Build history of the part. All positions in model axes, mm. A direction names the side the tool comes from. Round coordinates to 2 decimals unless told otherwise and drop trailing zeros. Write each loop counter-clockwise with the first axis right and the second up, starting at its lowest first coordinate (ties: lowest second). Pieces come first, ordered by that corner, then holes. Notation, with made-up numbers: (43, -12.5) -> (82, -12.5) arc R18 cw to (82, 11.5) -> close; hole circle Ø8 at (12.5, -2). An arc over 180 degrees is marked (long way). Answer in a Markdown table with one row per item. Add a question column.
from build123d import *

# Parameters (mm, degrees)
BOSS_EXTRUDE5_DEPTH      = 11
BOSS_EXTRUDE5_DEPTH_BACK = 5
SKETCH2_R                = 2.5


with BuildPart() as part:
    # Sketch1 → Revolve1 (revolve)
    with BuildSketch(Plane.XY, mode=Mode.PRIVATE) as revolve1_sk:
        Polygon((60, 80), (30, 80), (30, 40), (42.5, 40), (42.5, 0), (60, 0), align=None)
    revolve(revolve1_sk.sketch.rotate(Axis((30, 80, 0), (0, -1, 0)), 180), axis=Axis((30, 80, 0), (0, -1, 0)))

    # Sketch2 → Boss-Extrude5 (add, two sides: drawn at the far end of the back side and taken through both)
    with BuildSketch(Plane.XY.offset(-BOSS_EXTRUDE5_DEPTH_BACK)):
        with BuildLine():
            Line((46.5, 0), (46.5, -12))
            ThreePointArc((46.5, -12), (47.378679656, -14.121320344), (49.5, -15))
            Line((49.5, -15), (68.5, -15))
            ThreePointArc((68.5, -15), (70.621320344, -14.121320344), (71.5, -12))
            Line((71.5, -12), (71.5, -3))
            ThreePointArc((71.5, -3), (70.621320344, -0.878679656), (68.5, 0))
            Line((68.5, 0), (46.5, 0))
        make_face()
        with Locations((55, -8)):
            Circle(SKETCH2_R, mode=Mode.SUBTRACT)
    extrude(amount=BOSS_EXTRUDE5_DEPTH + BOSS_EXTRUDE5_DEPTH_BACK)


solid = part.part
(1) Saw through at A-A (y = -8). List the corners of the cut face in (x, z), plus the area to 3 significant figures.
(2) Drop flat-ended pins along their axis: P1, Ø16.5, axis at x = 60.5, y = -11, coming from the +Z side; P2, Ø4, axis at x = 59.5, z = -12.5, coming from the +Y side; P3, Ø3, axis at y = 38.5, z = -7.5, coming from the +X side; P4, Ø3, axis at x = 19, y = 25, coming from the +Z side. Give the stop position or say it passes through.
(3) Saw through at B-B (z = 0). List the corners of the cut face in (x, y), plus the area to 3 significant figures.
(4) Mould opens along Y. For faces 5 (the face through (57.31, -8.96, 2.89)), 6 (the face through (59, -7, 11)), 7 (the face through (30, 40, 0)) say: pulls with the +Y half, pulls with the -Y half, needs draft (parallel to the pull), parting line crosses it, or undercut.
(5) Probe line 1 along Y through (x, z) = (55, 1.5); line 2 along Z through (x, y) = (30, 31.5); line 3 along Z through (x, y) = (63, -0.5). List the from-to ranges inside material, lowest first.
(6) Which spindle directions (+Z, -Z, +X, -X, +Y, -Y) get a long thin tool onto all of the face, cutting with end or side? Do faces 1 (the face through (42.488, 19.72, -0.55)), 2 (the face through (46.5, -6, 3)), 3 (the face through (59, -7, -5)), 4 (the face through (70.6, -14.14, 2.89)). Say none if no direction does.
(7) Saw through at D-D (y = 11). List the corners of the cut face in (x, z), plus the area to 3 significant figures.
(8) Saw through at C-C (x = 30). List the corners of the cut face in (y, z).
Answer sheet:
| question | item | result |
|---|---|---|
| 1 | outline | (46.5, -5) -> (52.5, -5) -> (52.5, 11) -> (46.5, 11) -> close; (57.5, -5) -> (71.5, -5) -> (71.5, 11) -> (57.5, 11) -> close |
| 1 | area | 320 mm² |
| 2 | P1 | stops at z = 11 |
| 2 | P2 | passes through |
| 2 | P3 | stops at x = 59.39 |
| 2 | P4 | stops at z = 28.46 |
| 3 | outline | (0, 0) -> (17.5, 0) -> (17.5, 40) -> (42.5, 40) -> (42.5, 0) -> (46.5, 0) -> (46.5, -12) arc R3 ccw to (49.5, -15) -> (68.5, -15) arc R3 ccw to (71.5, -12) -> (71.5, -3) arc R3 ccw to (68.5, 0) -> (60, 0) -> (60, 80) -> (0, 80) -> close; hole circle Ø5 at (55, -8) |
| 3 | area | 4,150 mm² |
| 4 | face 5 | undercut |
| 4 | face 6 | needs draft |
| 4 | face 7 | pulls with the -Y half |
| 5 | line 1 | y = -15 to -10.5, -5.5 to 80 |
| 5 | line 2 | z = -30 to -12.5, 12.5 to 30 |
| 5 | line 3 | z = -5 to 11 |
| 6 | face 1 | -Y |
| 6 | face 2 | +Z, -Z, -X, -Y |
| 6 | face 3 | -Z, +X, -X, -Y |
| 6 | face 4 | +Z, -Z, +X, -Y |
| 7 | outline | circle Ø60 at (30, 0); hole circle Ø25 at (30, 0) |
| 7 | area | 2,340 mm² |
| 8 | outline | (0, -30) -> (80, -30) -> (80, 30) -> (0, 30) -> (0, 12.5) -> (40, 12.5) -> (40, -12.5) -> (0, -12.5) -> close |
